For this review, take the finished solid that the model builds, in its own axes (mm). A direction names the side the tool comes from. Coordinates: 2 decimals unless noted, no trailing zeros. Write each loop counter-clockwise with the first axis right and the second up, starting at its lowest first coordinate (ties: lowest second). Pieces come first, ordered by that corner, then holes.
```python
from build123d import *

# Parameters (mm, degrees)
F0_W      = 108.549212
F0_H      = 91.886736
F1_DEPTH  = 76.2
F2_W      = 92.835255
F2_H      = 78.426812
F3_DEPTH  = 82.55
F5_R      = 6.91847
F6_DEPTH  = 25.4
F7_W      = 48.028812
F7_H      = 25.447967
F8_DEPTH  = 25.4
F9_W      = 45.221382
F9_H      = 24.2807
F10_DEPTH = 25.4


with BuildPart() as f1:
    # F0 (on Top) → F1 (new body)
    with BuildSketch(Plane.XY):
        with Locations((6.926911, 2.629757)):
            Rectangle(F0_W, F0_H)
    extrude(amount=F1_DEPTH)

    # F2 (on Top) → F3 (cut)
    with BuildSketch(Plane.XY):
        with Locations((6.824679, 2.350463)):
            Rectangle(F2_W, F2_H)
    extrude(amount=F3_DEPTH, mode=Mode.SUBTRACT)

    # F5 (on face) → F6 (cut)
    with BuildSketch(Plane(origin=(-47.347695, 0, 0), x_dir=(0, -1, 0), z_dir=(-1, 0, 0))):
        with Locations((-17.136907, 53.27322)):
            Circle(F5_R)
    extrude(amount=-F6_DEPTH, mode=Mode.SUBTRACT)

    # F7 (on face) → F8 (cut)
    with BuildSketch(Plane.XZ.offset(43.313611)):
        with Locations((5.315581, 63.476017)):
            Rectangle(F7_W, F7_H)
    extrude(amount=-F8_DEPTH, mode=Mode.SUBTRACT)

    # F9 (on face) → F10 (cut)
    with BuildSketch(Plane(origin=(0, 48.573125, 0), x_dir=(-1, 0, 0), z_dir=(0, 1, 0))):
        with Locations((-9.750217, 64.05965)):
            Rectangle(F9_W, F9_H)
    extrude(amount=-F10_DEPTH, mode=Mode.SUBTRACT)


solid = f1.part
```
1) Clearance check with flat-ended pins moving along their axes: P1, Ø8.5, axis at y = 17.14, z = 53.27, coming from the -X side; P2, Ø2, axis at x = 2, y = 44.5, coming from the +Z side; P3, Ø3, axis at x = 7.5, y = -40, coming from the +Z side. State where each tip first meets the part, or that it passes through.
2) Tool access review of faces 4 (the face through (6, 41.564, 29)), 5 (the face through (32.361, 45, 64)), 6 (the face through (5, -40, 50.752)), 7 (the face through (-43.52, 13.42, 59.11)), 8 (the face through (-47.348, 2, 38)): name each direction out of +Z, -Z, +X, -X, +Y, -Y from which nothing blocks a thin tool from reaching the whole face with its end or side.
3) Consider section D-D (z = 35). Give the boundary of the cut face in (x, y), then the cut area to 3 significant figures.
4) For L1, parallel to Y at x = -19, z = 70.5; L2, parallel to X at y = -14, z = 39; L3, parallel to Y at x = -13, z = 56.5, list the stretches that pass through material, from the lowest coordinate up.
5) The part is to be moulded in two halves that separate along X. For faces 1 (the face through (61.202, 2, 38)), 2 (the face through (-12.86, 45, 64)), 3 (the face through (-42, 3, 76.2)), say which applies: pulls with the +X half, pulls with the -X half, needs draft (parallel to the pull), parting line crosses it, or undercut.
6) Consider section A-A (x = 12). Give the boundary of the cut face in (y, z), then the cut area to 3 significant figures.
7) Consider section C-C (y = 2). Give the boundary of the cut face in (x, z), then the cut area to 3 significant figures.
8) Consider section B-B (z = 71.5). Give the boundary of the cut face in (x, y), then the cut area to 3 significant figures.
Results:
1. P1: stops at x = 53.24
1. P2: stops at z = 51.92
1. P3: stops at z = 50.75
2. face 4: +Z, -Z
2. face 5: +Z, +Y
2. face 6: +Z, -Y
2. face 7: -X
2. face 8: +Z, -Z, -X, +Y, -Y
3. outline: (-47.35, -43.31) - (61.2, -43.31) - (61.2, 48.57) - (-47.35, 48.57) - close; hole (-39.59, -36.86) - (53.24, -36.86) - (53.24, 41.56) - (-39.59, 41.56) - close
3. area: 2,690 mm2
4. L1: y = -43.31 to -36.86, 41.56 to 48.57
4. L2: x = -47.35 to -39.59, 53.24 to 61.2
4. L3: y = 41.56 to 48.57
5. face 1: pulls with the +X half
5. face 2: undercut
5. face 3: needs draft
6. outline: (-43.31, 0) - (-36.86, 0) - (-36.86, 50.75) - (-43.31, 50.75) - close; (41.56, 0) - (48.57, 0) - (48.57, 51.92) - (41.56, 51.92) - close
6. area: 691 mm2
7. outline: (-47.35, 0) - (-39.59, 0) - (-39.59, 76.2) - (-47.35, 76.2) - close; (53.24, 0) - (61.2, 0) - (61.2, 76.2) - (53.24, 76.2) - close
7. area: 1,200 mm2
8. outline: (-47.35, -43.31) - (-18.7, -43.31) - (-18.7, -36.86) - (-39.59, -36.86) - (-39.59, 41.56) - (-12.86, 41.56) - (-12.86, 48.57) - (-47.35, 48.57) - close; (29.33, -43.31) - (61.2, -43.31) - (61.2, 48.57) - (32.36, 48.57) - (32.36, 41.56) - (53.24, 41.56) - (53.24, -36.86) - (29.33, -36.86) - close
8. area: 2,070 mm2
